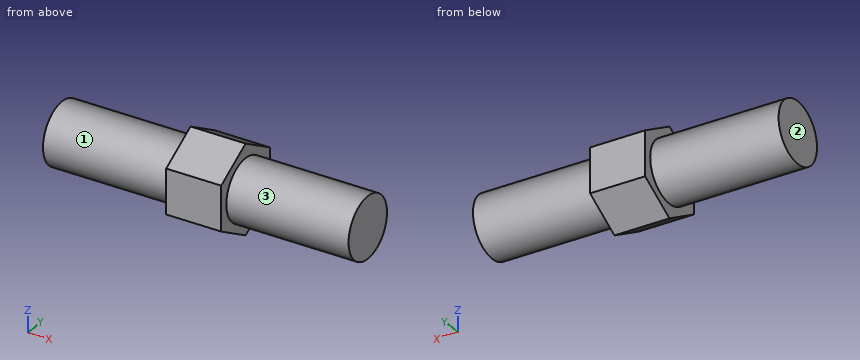
```python
from build123d import *

# Parameters (mm, degrees)
SKETCH1_W                = 15
SKETCH1_H                = 1.5
BOSS_EXTRUDE1_DEPTH      = 1.5
BOSS_EXTRUDE1_DEPTH_BACK = 1.2


with BuildPart() as part:
    # Sketch1 → Revolve1 (revolve)
    with BuildSketch(Plane(origin=(0, 0, 0), x_dir=(1, 0, 0), z_dir=(0, 1, 0)), mode=Mode.PRIVATE) as revolve1_sk:
        with Locations((0, 0.75)):
            Rectangle(SKETCH1_W, SKETCH1_H)
    revolve(revolve1_sk.sketch.rotate(Axis((-19.553100844, 0, 0), (1, 0, 0)), 180), axis=Axis((-19.553100844, 0, 0), (1, 0, 0)))

    # Sketch2 → Boss-Extrude1 (add, two sides: drawn at the far end of the back side and taken through both)
    with BuildSketch(Plane(origin=(0, 0, 0), x_dir=(0, 0, -1), z_dir=(1, 0, 0)).offset(-BOSS_EXTRUDE1_DEPTH_BACK)):
        Polygon((2.193931023, 0), (1.096965511, 1.9), (-1.096965511, 1.9), (-2.193931023, 0), (-1.096965511, -1.9), (1.096965511, -1.9), align=None)
    extrude(amount=BOSS_EXTRUDE1_DEPTH + BOSS_EXTRUDE1_DEPTH_BACK)


solid = part.part
```
The listing builds one solid part. Answer for the finished solid, in the listing's coordinates (mm). Face numbers are marked on the shaded views. A direction names the side the tool comes from. Coordinates: 2 decimals unless noted, no trailing zeros. Loops run counter-clockwise (first coordinate to the right, second up) from the corner with the lowest first, then second, coordinate; pieces in that order, holes last. Notation, with made-up numbers: M -26,-10 L -9,-10 A26 ccw -9,17 Z; hole C -37.75,26 d9. An arc over 180 degrees is marked long. Answer as a JSON object with one key per item and string values. Group by question number.
Item 1: Consider L1, parallel to X at y = 1.4, z = 0.7; L2, parallel to Y at x = -3.75, z = -0.1; L3, parallel to Z at x = 3, y = 1.25. Determine where each line is inside the solid, lowest interval first.
Item 2: Which of the six approach directions +Z, -Z, +X, -X, +Y, -Y give full straight-line access (tool end or side, diameter ignored) to the marked faces 1, 2 and 3?
Item 3: Section A-A (z = 0) is taken. Write down the section's boundary in (x, y).
Item 4: Section C-C (y = 1.1) is taken. Write down the section's boundary in (x, z).
Item 5: Each of these flat-tipped pins is pushed along its axis until it touches: P1, Ø1.5, axis at x = -2.5, z = 0, coming from the +Y side; P2, Ø1, axis at x = 5.5, y = 0.5, coming from the +Z side. Where does it stop, or does it pass through?
Item 6: Section B-B (x = -5.5) is taken. Write down the section's boundary in (y, z), and give its area (3 significant figures).
Solved:
{
 "1": {"L1": "x = -1.2 to 1.5", "L2": "y = -1.5 to 1.5", "L3": "z = -0.83 to 0.83"},
 "2": {"face 1": "-X", "face 2": "+Z, -Z, -X, +Y, -Y", "face 3": "+X"},
 "3": {"outline": "M -7.5,-1.5 L -1.2,-1.5 L -1.2,-1.9 L 1.5,-1.9 L 1.5,-1.5 L 7.5,-1.5 L 7.5,1.5 L 1.5,1.5 L 1.5,1.9 L -1.2,1.9 L -1.2,1.5 L -7.5,1.5 Z"},
 "4": {"outline": "M -7.5,-1.02 L -1.2,-1.02 L -1.2,-1.56 L 1.5,-1.56 L 1.5,-1.02 L 7.5,-1.02 L 7.5,1.02 L 1.5,1.02 L 1.5,1.56 L -1.2,1.56 L -1.2,1.02 L -7.5,1.02 Z"},
 "5": {"P1": "stops at y = 1.5", "P2": "stops at z = 1.5"},
 "6": {"outline": "C 0,0 d3", "area": "7.07 mm2"}
}
